from build123d import *

# Parameters (mm, degrees)
F0_R     = 0.75
F1_DEPTH = 15
F2_R     = 0.767857
F3_DEPTH = 4
F4_R     = 0.774571
F5_DEPTH = 4
F6_W     = 1.488906
F6_H     = 0.601098
F7_DEPTH = 2
F8_W     = 0.76025
F8_H     = 0.634269
F9_DEPTH = 25


with BuildPart() as f1:
    # F0 (on Top) → F1 (new body)
    with BuildSketch(Plane.XY):
        Circle(F0_R)
    extrude(amount=F1_DEPTH)

    # F2 (on Front) → F3 (join)
    with BuildSketch(Plane.XZ):
        with Locations((0, 4.209903)):
            Circle(F2_R)
    extrude(amount=F3_DEPTH)

    # F4 (on Front) → F5 (join)
    with BuildSketch(Plane.XZ):
        with Locations((0, 4.133399)):
            Circle(F4_R)
    extrude(amount=F5_DEPTH)

    # F6 (on Front) → F7 (join)
    with BuildSketch(Plane.XZ):
        with Locations((0, 6.574348)):
            Rectangle(F6_W, F6_H)
    extrude(amount=-F7_DEPTH)

    # F8 (on face) → F9 (cut)
    with BuildSketch(Plane(origin=(0, 0, 6.273799), x_dir=(1, 0, 0), z_dir=(0, 0, -1))):
        with Locations((0, -1.362656)):
            Rectangle(F8_W, F8_H)
    extrude(amount=-F9_DEPTH, mode=Mode.SUBTRACT)


solid = f1.part
Part model, mm, in its own coordinate system. A direction names the side the tool comes from. Coordinates: 2 decimals unless noted, no trailing zeros. Loops run counter-clockwise (first coordinate to the right, second up) from the corner with the lowest first, then second, coordinate; pieces in that order, holes last. Notation, with made-up numbers: (32, 16) - (69, 16) arc R9 ccw to (69, 26) - close; hole circle Ø5 at (3.25, -6.75). An arc over 180 degrees is marked (long way). Write each question's results on one line, items separated by ' | '. Start each with the question number.
Q1. Which spindle directions (+Z, -Z, +X, -X, +Y, -Y) get a long thin tool onto all of the face, cutting with end or side? Do faces 1 (the cylindrical face through (0.016, -2.416, 4.978)), 2 (the flat face through (0, 0, 0)), 3 (the cylindrical face through (-0.098, 0.744, 7.395)). Say none if no direction does.
Q2. Drop flat-ended pins along their axis: pin 1 Ø1.5 at (y, z) = (-0.5, 8.5) entering from -X; pin 2 Ø0.7 at (y, z) = (1.5, 6.5) entering from +X; pin 3 Ø0.7 at (x, y) = (0, 1.5) entering from +Z. Give the stop position or say it passes through.
Q3. Probe line 1 along Z through (x, y) = (-0.05, 1.75); line 2 along Y through (x, z) = (-0.1, 4.25); line 3 along Y through (x, z) = (0.1, 9.25). List the from-to ranges inside material, lowest first.
Q4. Slice it at B-B on z = 5.5. Give the cut face in (x, y).
Q5. Slice it at A-A on x = 0. Give the cut face in (y, z), and give its area (3 significant figures).
Answer:
1) face 1: +Z, -Y | face 2: -Z, +X, -X, +Y, -Y | face 3: none
2) pin 1: stops at x = -0.75 | pin 2: stops at x = 0.74 | pin 3: stops at z = 6.87
3) line 1: z = 6.27 to 6.87 | line 2: y = -4 to 0.74 | line 3: y = -0.74 to 0.74
4) outline: circle Ø1.5 at (0, 0)
5) outline: (-4, 3.36) - (-0.75, 3.36) - (-0.75, 0) - (0.75, 0) - (0.75, 6.27) - (1.05, 6.27) - (1.05, 6.87) - (0.75, 6.87) - (0.75, 15) - (-0.75, 15) - (-0.75, 4.98) - (-4, 4.98) - close; (1.68, 6.27) - (2, 6.27) - (2, 6.87) - (1.68, 6.87) - close | area: 28.1 mm2
